The drawing under review shows one solid part. Ordinate dimensions are in mm from its lowest x, y, z. A direction names the side the tool comes from. Give positions to 0.01 mm unless a question says otherwise; leave off trailing zeros. Order: outer loops, then holes, each group sorted by start corner. A loop starts at its lowest first (then second) coordinate and runs counter-clockwise, first axis right, second up. Notation, with made-up numbers: (15.25, 25) - (27.25, 25) arc R10 cw to (27.25, 36) - close; hole circle Ø3 at (17.25, -34). An arc over 180 degrees is marked (long way). Use CSV: the item, a comma, the result in double quotes. Start each with the question number.
1. Draft analysis for pull direction X (two halves, no side actions). For the marked faces 3, 4, 5 and 6, state which applies: released by +X, released by -X, zero draft, split by the parting line, or undercut.
2. Take a section at C-C, the plane x = 8. State the section outline as (y, z) points.
3. Take a section at A-A, the plane z = 19.05. State the section outline as (x, y) points, then the cut area to 3 significant figures.
4. Machinability: for the marked faces 1 and 2, which of the approach directions +Z, -Z, +X, -X, +Y, -Y give a long, thin tool a straight path to every point of the face, cutting with its end or side? Answer none if there is none.
5. Take a section at B-B, the plane x = 31.75. State the section outline as (y, z) points, then the cut area to 3 significant figures.
6. For pin 1 (16 mm diameter, centred on x = 30.5, y = 22, fed in from +Z); pin 2 (12 mm diameter, centred on y = 15, z = 26, fed in from +X), all flat-tipped, find the tip position at first contact; note any pin that passes through.
7. To check wall thickness, follow line 1 (X direction, y = 18.5, z = 6.35); line 2 (X direction, y = 13, z = 19); line 3 (X direction, y = 18, z = 8). State the ranges of each line that lie inside material, in increasing order. Write a range as [from, to].
8. Take a section at D-D, the plane y = 9. Count the separate pieces of the cut face and the enclosed holes in it.
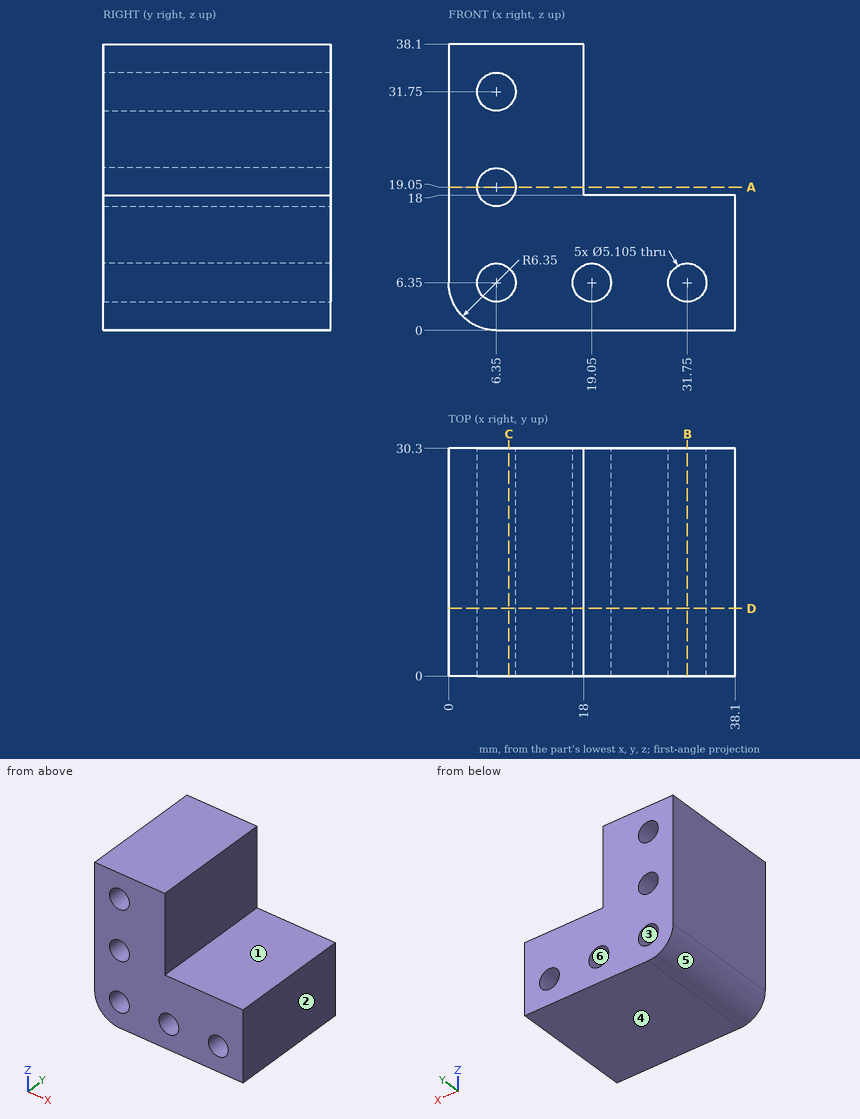
Determined:
1,face 3,"undercut"
1,face 4,"zero draft"
1,face 5,"released by -X"
1,face 6,"undercut"
2,outline,"(0, 0) - (30.3, 0) - (30.3, 4.4) - (0, 4.4) - close; (0, 8.3) - (30.3, 8.3) - (30.3, 17.1) - (0, 17.1) - close; (0, 21) - (30.3, 21) - (30.3, 29.8) - (0, 29.8) - close; (0, 33.7) - (30.3, 33.7) - (30.3, 38.1) - (0, 38.1) - close"
3,outline,"(0, 0) - (3.8, 0) - (3.8, 30.3) - (0, 30.3) - close; (8.9, 0) - (18, 0) - (18, 30.3) - (8.9, 30.3) - close"
3,area,"391 mm²"
4,face 1,"+Z, +X, +Y, -Y"
4,face 2,"+Z, -Z, +X, +Y, -Y"
5,outline,"(0, 0) - (30.3, 0) - (30.3, 3.8) - (0, 3.8) - close; (0, 8.9) - (30.3, 8.9) - (30.3, 18) - (0, 18) - close"
5,area,"391 mm²"
6,pin 1,"stops at z = 18"
6,pin 2,"stops at x = 18"
7,line 1,"x = [0, 3.8], [8.9, 16.5], [21.6, 29.2], [34.3, 38.1]"
7,line 2,"x = [0, 3.8], [8.9, 18]"
7,line 3,"x = [0, 4.4], [8.3, 17.1], [21, 29.8], [33.7, 38.1]"
8,separate pieces,"1"
8,enclosed holes,"5"
